Job drawing, mm, ordinate dimensions from the low corner. One solid piece. A direction names the side the tool comes from. Round coordinates to 2 decimals unless told otherwise and drop trailing zeros. Order: outer loops, then holes, each group sorted by start corner. A loop starts at its lowest first (then second) coordinate and runs counter-clockwise, first axis right, second up. Notation, with made-up numbers: (41.5, 46.25) -> (75.5, 46.25) arc R21 ccw to (75.5, 60.25) -> close; hole circle Ø9 at (13, 24). An arc over 180 degrees is marked (long way). Answer as a JSON object with one key per item and string values. Group by question number.
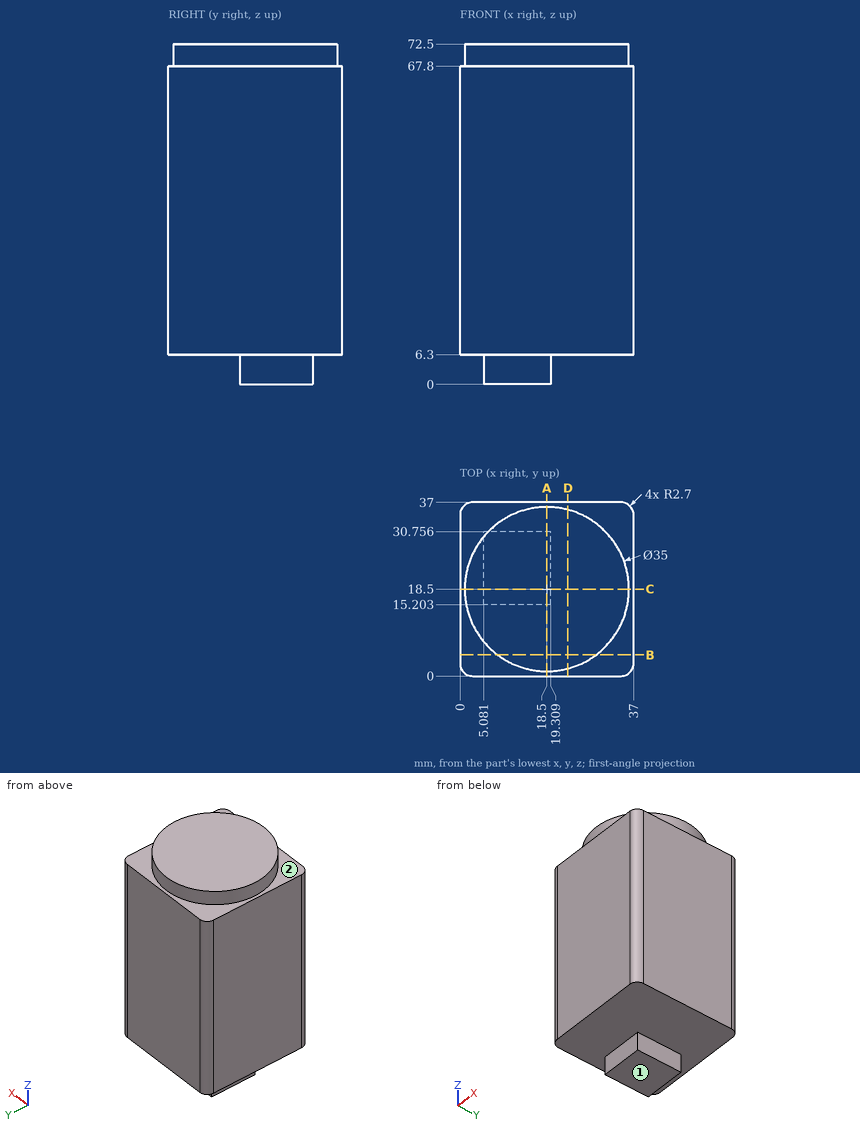
Q1. Band-saw the part on D-D (x = 23). List the corners of the cut face in (y, z), plus the area to 3 significant figures.
Q2. Drop flat-ended pins along their axis: pin 1 Ø12 at (x, y) = (33, 26) entering from -Z; pin 2 Ø3 at (x, z) = (15, 2.5) entering from +Y; pin 3 Ø7 at (y, z) = (24, 2) entering from -X. Give the stop position or say it passes through.
Q3. Wall check: line 1 (Z direction, x = 26, y = 27.5); line 2 (Y direction, x = 2.5, z = 49.5); line 3 (X direction, y = 17, z = 5). Give the ranges that are in metal, low to high. Write a range as [from, to].
Q4. Band-saw the part on C-C (y = 18.5). List the corners of the cut face in (x, z), plus the area to 3 significant figures.
Q5. Which spindle directions (+Z, -Z, +X, -X, +Y, -Y) get a long thin tool onto all of the face, cutting with end or side? Do the marked faces 1 and 2. Say none if no direction does.
Q6. Band-saw the part on B-B (y = 4.5). List the corners of the cut face in (x, z), plus the area to 3 significant figures.
Q7. Band-saw the part on A-A (x = 18.5). List the corners of the cut face in (y, z), plus the area to 3 significant figures.
Completed:
{
 "1": {"outline": "(0, 6.3) -> (37, 6.3) -> (37, 67.8) -> (35.41, 67.8) -> (35.41, 72.5) -> (1.59, 72.5) -> (1.59, 67.8) -> (0, 67.8) -> close", "area": "2,430 mm2"},
 "2": {"pin 1": "z = 6.3", "pin 2": "y = 30.76", "pin 3": "x = 5.08"},
 "3": {"line 1": "[6.3, 72.5]", "line 2": "[0.01, 36.99]", "line 3": "[5.08, 19.31]"},
 "4": {"outline": "(0, 6.3) -> (5.08, 6.3) -> (5.08, 0) -> (19.31, 0) -> (19.31, 6.3) -> (37, 6.3) -> (37, 67.8) -> (36, 67.8) -> (36, 72.5) -> (1, 72.5) -> (1, 67.8) -> (0, 67.8) -> close", "area": "2,530 mm2"},
 "5": {"face 1": "-Z, +X, -X, +Y, -Y", "face 2": "+Z"},
 "6": {"outline": "(0, 6.3) -> (37, 6.3) -> (37, 67.8) -> (29, 67.8) -> (29, 72.5) -> (8, 72.5) -> (8, 67.8) -> (0, 67.8) -> close", "area": "2,370 mm2"},
 "7": {"outline": "(0, 6.3) -> (15.2, 6.3) -> (15.2, 0) -> (30.76, 0) -> (30.76, 6.3) -> (37, 6.3) -> (37, 67.8) -> (36, 67.8) -> (36, 72.5) -> (1, 72.5) -> (1, 67.8) -> (0, 67.8) -> close", "area": "2,540 mm2"}
}
